Check sheet for the modelled part. Datum: model origin and axes. Units: mm. Face numbers are marked on the shaded views. A direction names the side the tool comes from. Round coordinates to 2 decimals unless told otherwise and drop trailing zeros. Loops run counter-clockwise (first coordinate to the right, second up) from the corner with the lowest first, then second, coordinate; pieces in that order, holes last. Notation, with made-up numbers: (-4, 61) - (50, 61) arc R22 cw to (50, 72) - close; hole circle Ø10 at (-23.75, -16). An arc over 180 degrees is marked (long way). Put each result on its own line as item: value. Start each with the question number.
```python
from build123d import *

# Parameters (mm, degrees)
SKETCH2_W           = 70
SKETCH2_H           = 39.7
BOSS_EXTRUDE1_DEPTH = 1.7
BOSS_EXTRUDE2_DEPTH = 8
SKETCH6_W           = 60
SKETCH6_H           = 10.2
BOSS_EXTRUDE3_DEPTH = 3
SKETCH7_W           = 44.8
SKETCH7_H           = 6.5
BOSS_EXTRUDE4_DEPTH = 20.8
CUT_EXTRUDE1_REACH  = 60.08
SKETCH8_W           = 22.5
SKETCH8_H           = 12.8
CUT_EXTRUDE2_REACH  = 60.08
SKETCH9_R           = 1
CUT_EXTRUDE3_REACH  = 52.49
SKETCH10_R          = 1.5
SKETCH13_W          = 60
SKETCH13_H          = 5.5
CUT_EXTRUDE4_DEPTH  = 4.5
SKETCH14_W          = 60
SKETCH14_H          = 5.5
CUT_EXTRUDE5_DEPTH  = 4.5


with BuildPart() as part:
    # Sketch2 → Boss-Extrude1 (new body)
    with BuildSketch(Plane(origin=(0, 0, 0), x_dir=(1, 0, 0), z_dir=(0, 1, 0))):
        Rectangle(SKETCH2_W, SKETCH2_H)
    extrude(amount=BOSS_EXTRUDE1_DEPTH)

    # Sketch3 → Boss-Extrude2 (add)
    with BuildSketch(Plane(origin=(0, 1.7, 0), x_dir=(1, 0, 0), z_dir=(0, 1, 0))):
        Polygon((35, 15.05), (-29.6, 15.05), (-29.6, -14.45), (35, -14.45), (35, -4.95), (-25, -4.95), (-25, 5.25), (35, 5.25), align=None)
    extrude(amount=BOSS_EXTRUDE2_DEPTH)

    # Sketch6 → Boss-Extrude3 (add)
    with BuildSketch(Plane(origin=(0, 1.7, 0), x_dir=(1, 0, 0), z_dir=(0, 1, 0))):
        with Locations((5, 0.15)):
            Rectangle(SKETCH6_W, SKETCH6_H)
    extrude(amount=BOSS_EXTRUDE3_DEPTH)

    # Sketch7 → Boss-Extrude4 (add)
    with BuildSketch(Plane(origin=(0, 9.7, 0), x_dir=(1, 0, 0), z_dir=(0, 1, 0))):
        with Locations((2.6, 11.8)):
            Rectangle(SKETCH7_W, SKETCH7_H)
    extrude(amount=BOSS_EXTRUDE4_DEPTH)

    # Sketch8 → Cut-Extrude1 (cut, up to next)
    with BuildSketch(Plane(origin=(0, 0, -15.05), x_dir=(-1, 0, 0), z_dir=(0, 0, -1)), mode=Mode.PRIVATE) as cut_extrude1_sk1:
        with Locations((-1.95, 21.3)):
            Rectangle(SKETCH8_W, SKETCH8_H)
    cut_extrude1_tool1 = extrude(cut_extrude1_sk1.sketch, amount=-CUT_EXTRUDE1_REACH, mode=Mode.PRIVATE) & part.part
    add(cut_extrude1_tool1.solids().sort_by_distance((1.95, 21.3, -15.05))[0], mode=Mode.SUBTRACT)

    # Sketch9 → Cut-Extrude2 (cut, up to next)
    with BuildSketch(Plane(origin=(0, 0, -15.05), x_dir=(-1, 0, 0), z_dir=(0, 0, -1)), mode=Mode.PRIVATE) as cut_extrude2_sk1:
        with Locations((-15.7, 21.3)):
            Circle(SKETCH9_R)
    cut_extrude2_tool1 = extrude(cut_extrude2_sk1.sketch, amount=-CUT_EXTRUDE2_REACH, mode=Mode.PRIVATE) & part.part
    # Sketch9 → Cut-Extrude2 (cut, up to next)
    with BuildSketch(Plane(origin=(0, 0, -15.05), x_dir=(-1, 0, 0), z_dir=(0, 0, -1)), mode=Mode.PRIVATE) as cut_extrude2_sk2:
        with Locations((11.8, 21.3)):
            Circle(SKETCH9_R)
    cut_extrude2_tool2 = extrude(cut_extrude2_sk2.sketch, amount=-CUT_EXTRUDE2_REACH, mode=Mode.PRIVATE) & part.part
    add(cut_extrude2_tool1.solids().sort_by_distance((15.7, 21.3, -15.05))[0], mode=Mode.SUBTRACT)
    add(cut_extrude2_tool2.solids().sort_by_distance((-11.8, 21.3, -15.05))[0], mode=Mode.SUBTRACT)

    # Sketch10 → Cut-Extrude3 (cut, up to next)
    with BuildSketch(Plane.XZ, mode=Mode.PRIVATE) as cut_extrude3_sk1:
        with Locations(Location((-32.5, 17.35, 0), (0, 0, 270))):
            Circle(SKETCH10_R)
    cut_extrude3_tool1 = extrude(cut_extrude3_sk1.sketch, amount=-CUT_EXTRUDE3_REACH, mode=Mode.PRIVATE) & part.part
    # Sketch10 → Cut-Extrude3 (cut, up to next)
    with BuildSketch(Plane.XZ, mode=Mode.PRIVATE) as cut_extrude3_sk2:
        with Locations(Location((32.5, 17.35, 0), (0, 0, 270))):
            Circle(SKETCH10_R)
    cut_extrude3_tool2 = extrude(cut_extrude3_sk2.sketch, amount=-CUT_EXTRUDE3_REACH, mode=Mode.PRIVATE) & part.part
    cut_extrude3_1 = cut_extrude3_tool1.solids().sort_by_distance((-32.5, 0, 17.35))[0]
    add(cut_extrude3_1, mode=Mode.SUBTRACT)
    cut_extrude3_2 = cut_extrude3_tool2.solids().sort_by_distance((32.5, 0, 17.35))[0]
    add(cut_extrude3_2, mode=Mode.SUBTRACT)
    cut_extrude3 = cut_extrude3_1 + cut_extrude3_2  # Cut-Extrude3 as one shape, for the pattern or mirror that repeats it

    # Mirror1: Cut-Extrude3 across plane
    add(cut_extrude3.mirror(Plane.XY), mode=Mode.SUBTRACT)

    # Sketch13 → Cut-Extrude4 (cut)
    with BuildSketch(Plane.XZ):
        with Locations((2.2, -10.6)):
            Rectangle(SKETCH13_W, SKETCH13_H)
    extrude(amount=-CUT_EXTRUDE4_DEPTH, mode=Mode.SUBTRACT)

    # Sketch14 → Cut-Extrude5 (cut)
    with BuildSketch(Plane.XZ):
        with Locations((2.5, 10.1)):
            Rectangle(SKETCH14_W, SKETCH14_H)
    extrude(amount=-CUT_EXTRUDE5_DEPTH, mode=Mode.SUBTRACT)


solid = part.part
```
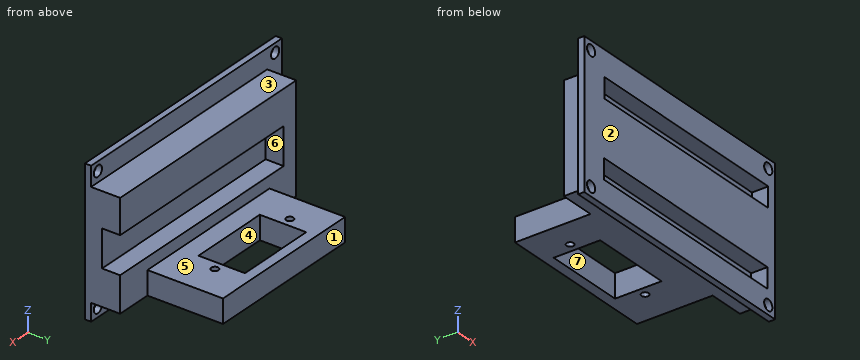
Q1. Cross-section at A-A on x = -32.5. Enter the section's corners in (y, z), and give its area (3 significant figures).
Q2. Set-up check for the marked faces 5, 6 and 7: record each of +Z, -Z, +X, -X, +Y, -Y from which the full face is reachable in a straight line by a thin tool's end or side.
Q3. Material ranges on line 1 (Z direction, x = 21, y = 3); line 2 (X direction, y = 0.5, z = -17.35); line 3 (Z direction, x = -14.5, y = 1), recorded low to high. Write a range as from..to.
Q4. Depth check by flat-ended pin: pin 1 Ø2.5 at (x, y) = (15.7, 21.3) entering from +Z; pin 2 Ø8 at (x, z) = (14, 11.5) entering from -Y; pin 3 Ø6 at (x, z) = (-27, -9) entering from +Y; pin 4 Ø1.6 at (x, z) = (-12.5, -12) entering from -Y. Enter the tip coordinate at first touch or a pass-through.
Q5. Cross-section at C-C on x = -7. Enter the section's corners in (y, z), and give its area (3 significant figures).
Q6. Cross-section at D-D on y = 21.3. Enter the section's corners in (x, z).
Q7. Draft check along Y on the marked faces 1, 2, 3 and 4. Enter one of: +Y half, -Y half, draft (parallel to the pull), parting line (faces both ways), or undercut.
Q8. Cross-section at B-B on z = -17.35. Enter the section's corners in (x, y).
Answer list:
1. outline: (0, -19.85) - (1.7, -19.85) - (1.7, -18.85) - (0, -18.85) - close; (0, -15.85) - (1.7, -15.85) - (1.7, 15.85) - (0, 15.85) - close; (0, 18.85) - (1.7, 18.85) - (1.7, 19.85) - (0, 19.85) - close
1. area: 57.3 mm2
2. face 5: +Z, +X, -X, +Y
2. face 6: +X, +Y
2. face 7: +Z, -Z
3. line 1: z = -15.05..-13.35, -7.85..7.35, 12.85..14.45
3. line 2: x = -35..-34, -31..31, 34..35
3. line 3: z = -19.85..-13.35, -7.85..7.35, 12.85..19.85
4. pin 1: stops at z = -8.55
4. pin 2: stops at y = 0
4. pin 3: stops at y = 9.7
4. pin 4: stops at y = 4.5
5. outline: (0, -19.85) - (1.7, -19.85) - (1.7, -15.05) - (14.9, -15.05) - (14.9, -8.55) - (9.7, -8.55) - (9.7, -5.25) - (4.7, -5.25) - (4.7, 4.95) - (9.7, 4.95) - (9.7, 14.45) - (1.7, 14.45) - (1.7, 19.85) - (0, 19.85) - (0, 12.85) - (4.5, 12.85) - (4.5, 7.35) - (0, 7.35) - (0, -7.85) - (4.5, -7.85) - (4.5, -13.35) - (0, -13.35) - close; (27.7, -15.05) - (30.5, -15.05) - (30.5, -8.55) - (27.7, -8.55) - close
5. area: 255 mm2
6. outline: (-19.8, -15.05) - (-12.8, -15.05) - (-12.8, -8.55) - (-19.8, -8.55) - close; (-10.8, -15.05) - (-9.3, -15.05) - (-9.3, -8.55) - (-10.8, -8.55) - close; (13.2, -15.05) - (14.7, -15.05) - (14.7, -8.55) - (13.2, -8.55) - close; (16.7, -15.05) - (25, -15.05) - (25, -8.55) - (16.7, -8.55) - close
7. face 1: +Y half
7. face 2: -Y half
7. face 3: draft
7. face 4: undercut
8. outline: (-35, 0) - (-34, 0) - (-34, 1.7) - (-35, 1.7) - close; (-31, 0) - (31, 0) - (31, 1.7) - (-31, 1.7) - close; (34, 0) - (35, 0) - (35, 1.7) - (34, 1.7) - close
